Autodesk Inventor part; units mm, degrees
ref_plane "YZ Plane" through (0, 0, 0) normal (1, 0, 0) x (0, 1, 0)
ref_plane "XZ Plane" through (0, 0, 0) normal (0, 1, 0) x (-1, 0, 0)
ref_plane "XY Plane" through (0, 0, 0) normal (0, 0, 1) x (1, 0, 0)
sketch "スケッチ1" plane through (0, 0, 0) normal (0, 0, 1) x (1, 0, 0)
  line L0 (-120, 75) -> (120, 75)
  line L1 (120, 75) -> (120, -75)
  line L2 (120, -75) -> (-120, -75)
  line L3 (-120, -75) -> (-120, 75)
  line L4 (-120, 75) -> (120, -75) construction
  line L5 (120, 75) -> (-120, -75) construction
  point P0 (0, 0)
  dimension "d0" = 240
  dimension "d1" = 150
extrude "押し出し1" add sketch "スケッチ1" along normal blind 1.5
sketch "スケッチ2" plane through (0, 0, 1.5) normal (0, 0, 1) x (1, 0, 0)
  line L0 (-120, 75) -> (-120, -75)
  line L1 (120, 75) -> (-120, 75)
  line L2 (-120, -75) -> (120, -75)
  point P0 (0, 0)
  point P1 (-70, 21.25)
  point P2 (-70, -21.25)
  point P3 (40, 21.25)
  point P4 (40, -21.25)
  point P5 (55, 21.25)
  point P6 (55, -21.25)
  point P7 (-115, 30)
  point P8 (-115, -30)
  dimension "d4" = 50
  dimension "d5" = 53.75
  dimension "d6" = 50
  dimension "d7" = 53.75
  dimension "d8" = 160
  dimension "d9" = 53.75
  dimension "d10" = 53.75
  dimension "d11" = 15
  dimension "d12" = 15
  dimension "d13" = 53.75
  dimension "d14" = 53.75
  dimension "d22" = 60
  dimension "d23" = 30
  dimension "d24" = 5
  dimension "d42" = 42.5
hole "穴1" at (-70, 21.25, 1.5) at (-70, -21.25, 1.5) at (40, 21.25, 1.5) at (40, -21.25, 1.5) at (55, 21.25, 1.5) at (55, -21.25, 1.5) at (-115, 30, 1.5) at (-115, -30, 1.5) direction (0, 0, -1) diameter 3.1 end through all
sketch "スケッチ4" plane through (0, 0, 1.5) normal (0, 0, 1) x (1, 0, 0)
  line L0 (-120, 75) -> (-120, -75)
  point P0 (0, 0)
  point P1 (25, 50)
  point P2 (25, -50)
  point P3 (75, 50)
  point P4 (75, -50)
  dimension "d25" = 195
  dimension "d26" = 195
  dimension "d27" = 145
  dimension "d28" = 145
  dimension "d29" = 100
  dimension "d30" = 100
  dimension "d33" = 50
  dimension "d34" = 50
hole "穴2" at (25, 50, 1.5) at (25, -50, 1.5) at (75, 50, 1.5) at (75, -50, 1.5) direction (0, 0, -1) diameter 3.1 depth 3.2 tip angle 118
sketch "スケッチ5" plane through (0, 0, 1.5) normal (0, 0, 1) x (1, 0, 0)
  line L0 (-120, -75) -> (120, -75)
  line L1 (120, 75) -> (80, 75)
  line L2 (80, 75) -> (80, -75)
  line L3 (80, -75) -> (120, -75)
  line L4 (120, -75) -> (120, 75)
  point P0 (0, 0)
  dimension "d43" = 40
extrude "押し出し2" cut sketch "スケッチ5" against normal blind 10
sketch "スケッチ6" plane through (0, 0, 1.5) normal (0, 0, 1) x (1, 0, 0)
  line L0 (-120, -75) -> (80, -75)
  line L1 (80, -75) -> (80, -65)
  line L2 (80, -65) -> (-120, -65)
  line L3 (-120, -65) -> (-120, -75)
  line L4 (-120, 75) -> (80, 75)
  line L5 (80, 75) -> (80, 65)
  line L6 (80, 65) -> (-120, 65)
  line L7 (-120, 65) -> (-120, 75)
  point P0 (0, 0)
  dimension "d46" = 200
  dimension "d47" = 10
  dimension "d48" = 200
  dimension "d49" = 10
extrude "押し出し3" cut sketch "スケッチ6" against normal blind 10
sketch "スケッチ7" plane through (0, 0, 1.5) normal (0, 0, 1) x (1, 0, 0)
  circle A0 centre (-25, 0) radius 7.5
  point P0 (0, 0)
  dimension "d52" = 15
  dimension "d55" = 25
extrude "押し出し4" cut sketch "スケッチ7" against normal blind 10
fillet "フィレット1" radius 10 4 edges at (80, -65, 0.75) (80, 65, 0.75) (-120, 65, 0.75) (-120, -65, 0.75)
sketch "スケッチ8" plane through (0, 0, 1.5) normal (0, 0, 1) x (1, 0, 0)
  line L0 (-110, -65) -> (70, -65)
  line L1 (70, 65) -> (-110, 65)
  circle A0 centre (25, 50) radius 1.55
  line L2 (80, -55) -> (80, 55)
  point P0 (0, 0)
  point P1 (-57, -46)
  point P2 (15, -46)
  point P3 (-57, 46)
  point P4 (15, 46)
  dimension "d59" = 19
  dimension "d60" = 19
  dimension "d61" = 72
  dimension "d64" = 65
hole "穴3" at (-57, -46, 1.5) at (15, -46, 1.5) at (-57, 46, 1.5) at (15, 46, 1.5) direction (0, 0, -1) diameter 3.2 end through all
properties part number "Board 2" material "アルミニウム 6061"
CAD build for the part. Positions are in the model's coordinates, mm. Round coordinates to 2 decimals unless told otherwise and drop trailing zeros. Write each loop counter-clockwise with the first axis right and the second up, starting at its lowest first coordinate (ties: lowest second). Pieces come first, ordered by that corner, then holes. Notation, with made-up numbers: M -10.5,51 L 12.5,51 A34 ccw 12.5,85 Z; hole C -24,53.5 d5. An arc over 180 degrees is marked long. Put each result on its own line as item: value. Start each with the question number.
1) Saw through at B-B, the plane y = 0. Write the cut outline in (x, z), and give its area (4 significant figures).
2) Pull direction X, two halves, no side cores. Call faces 1 (the cylindrical face through (-117.15, 61.99, 0.74)), 2 (the cylindrical face through (-32.493, 0.33, 0.76)), 3 (the flat face through (-21, 15, 1.5)): pulls with the +X half, pulls with the -X half, needs draft (parallel to the pull), parting line crosses it, or undercut.
3) Saw through at A-A, the plane x = -25. Write the cut outline in (y, z).
4) Drill centre lines: probe 1 along Y at (x, z) = (-57, 0.6); probe 2 along X at (y, z) = (-46, 0.6); probe 3 along X at (y, z) = (50, 1). Where is each one in solid material? Low to high. Write a range as [from, to].
Resolved:
1. outline: M -120,0 L -32.5,0 L -32.5,1.5 L -120,1.5 Z; M -17.5,0 L 80,0 L 80,1.5 L -17.5,1.5 Z
1. area: 277.5 mm²
2. face 1: pulls with the -X half
2. face 2: undercut
2. face 3: needs draft
3. outline: M -65,0 L -7.5,0 L -7.5,1.5 L -65,1.5 Z; M 7.5,0 L 65,0 L 65,1.5 L 7.5,1.5 Z
4. probe 1: [-65, -47.6], [-44.4, 44.4], [47.6, 65]
4. probe 2: [-120, -58.6], [-55.4, 13.4], [16.6, 80]
4. probe 3: [-120, 23.45], [26.55, 73.45], [76.55, 80]
